Geometry: see drawing. Coordinates: mm, zero at the bounding-box minimum. A direction names the side the tool comes from. Give positions to 0.01 mm unless a question says otherwise; leave off trailing zeros. Loops run counter-clockwise (first coordinate to the right, second up) from the corner with the lowest first, then second, coordinate; pieces in that order, holes last. Notation, with made-up numbers: M 13.25,-33 L 41.25,-33 A21 cw 41.25,-23 Z; hole C 17.25,1.5 d3. An arc over 180 degrees is marked long. Put each result on its own line as item: value.
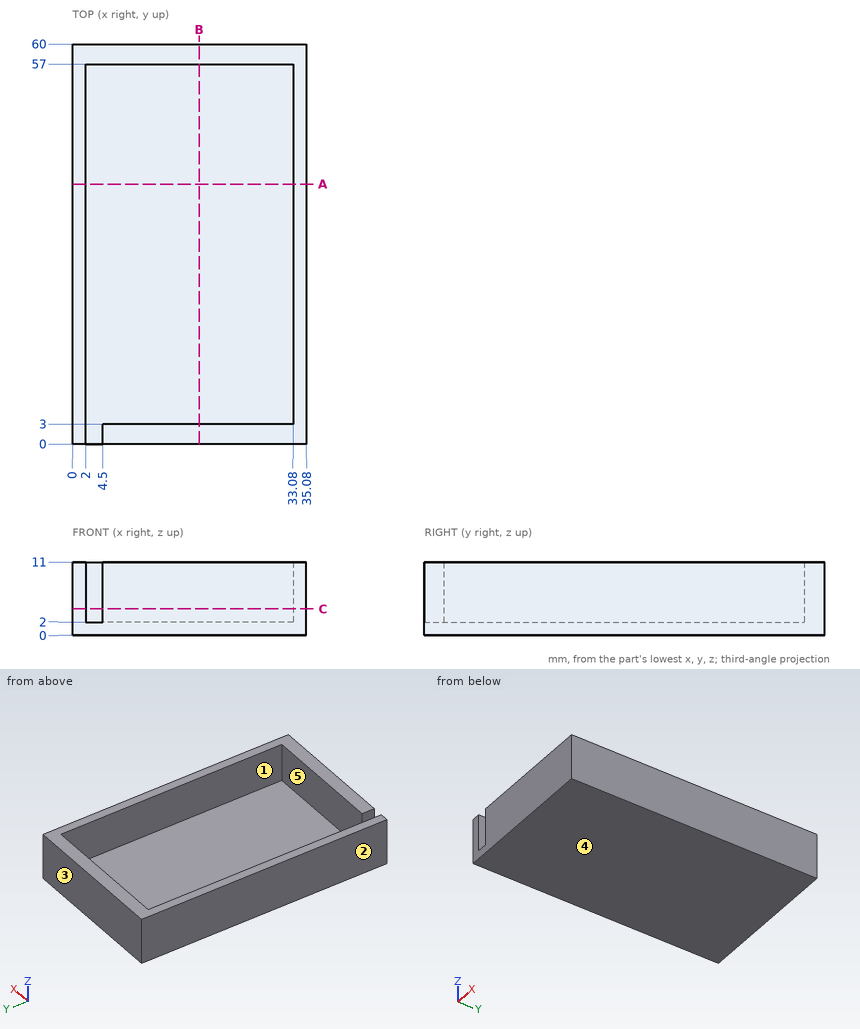
1. Section query C-C (z = 4). Output: boundary loops of the cut face in (x, y).
Found:
outline: M 0,0 L 2,0 L 2,57 L 33.08,57 L 33.08,3 L 4.5,3 L 4.5,0 L 35.08,0 L 35.08,60 L 0,60 Z
2. Draft query along Y for the marked faces 1, 2 and 3. Return one class per face: pulls with the +Y half, pulls with the -Y half, needs draft (parallel to the pull), parting line crosses it, or undercut.
Found:
face 1: undercut
face 2: needs draft
face 3: pulls with the +Y half
3. Contact query for flat-ended pins moving along their axis: P1, Ø3.5, axis at y = 1, z = 4.5, coming from the -X side; P2, Ø8, axis at x = 26.5, y = 23.5, coming from the +Z side. Output: stop coordinate, or through.
Found:
P1: x = 0
P2: z = 2
4. Access query for the marked faces 4 and 5. Directions: +Z, -Z, +X, -X, +Y, -Y. A direction counts if a zero-diameter tool reaches every point of the face in a straight line with its end or side. Return the directions, or none.
Found:
face 4: -Z, +X, -X, +Y, -Y
face 5: +Z
5. Section query A-A (y = 39). Output: boundary loops of the cut face in (x, z).
Found:
outline: M 0,0 L 35.08,0 L 35.08,11 L 33.08,11 L 33.08,2 L 2,2 L 2,11 L 0,11 Z
6. Section query B-B (x = 19). Output: boundary loops of the cut face in (y, z), plus the area to 3 significant figures.
Found:
outline: M 0,0 L 60,0 L 60,11 L 57,11 L 57,2 L 3,2 L 3,11 L 0,11 Z
area: 174 mm^2
7. Material intervals for line 1 (Y direction, x = 31.5, z = 8.25); line 2 (X direction, y = 37, z = 8.75); line 3 (Z direction, x = 33, y = 10), sorted ascending. Write a range as from..to.
Found:
line 1: 0..3, 57..60
line 2: 0..2, 33.08..35.08
line 3: 0..2
